Build history of the part. All positions in model axes, mm. Round coordinates to 2 decimals unless told otherwise and drop trailing zeros. Write each loop counter-clockwise with the first axis right and the second up, starting at its lowest first coordinate (ties: lowest second). Pieces come first, ordered by that corner, then holes. Notation, with made-up numbers: M -38.75,85.25 L -8.75,85.25 A18 cw -8.75,94.25 Z; hole C -28,3 d9. An arc over 180 degrees is marked long. Use a Markdown table: item, result.
Autodesk Inventor part; units mm, degrees
ref_plane "YZ Plane" through (0, 0, 0) normal (1, 0, 0) x (0, 1, 0)
ref_plane "XZ Plane" through (0, 0, 0) normal (0, 1, 0) x (-1, 0, 0)
ref_plane "XY Plane" through (0, 0, 0) normal (0, 0, 1) x (1, 0, 0)
sketch "Sketch1" plane through (0, 0, 0) normal (0, 0, 1) x (1, 0, 0)
  line L0 (0, 40) -> (0, 0)
  line L1 (0, 0) -> (6, 0)
  line L2 (6, 0) -> (6, 8)
  line L3 (6, 8) -> (22, 8)
  line L4 (22, 8) -> (22, 0)
  line L5 (22, 0) -> (28, 0)
  line L6 (28, 0) -> (28, 40)
  line L7 (28, 40) -> (0, 40)
  dimension "d0" = 6
  dimension "d1" = 6
  dimension "d2" = 16
  dimension "d3" = 40
  dimension "d4" = 8
extrude "Extrusion1" add sketch "Sketch1" against normal blind 8
sketch "Sketch2" plane through (28, 0, 0) normal (1, 0, 0) x (0, 0, -1)
  circle A0 centre (4, 4) radius 2
  line L0 (0, 0) -> (8, 0)
  line L1 (0, 0) -> (8, 0)
  point P0 (4, 0)
  dimension "d7" = 4
  dimension "d8" = 4
  dimension "d9" = 8
extrude "Extrusion2" cut sketch "Sketch2" against normal through all
fillet "Fillet1" radius 4 5 edges at (25, 0, 0) (3, 0, 0) (3, 0, -8) (25, 0, -8) (14, 8, -8)
sketch "Sketch3" plane through (0, 0, -8) normal (0, 0, -1) x (-1, 0, 0)
  line L0 (0, 40) -> (-28, 40)
  line L1 (-20, 40) -> (-16, 40)
  line L2 (-16, 40) -> (-16, 32)
  line L3 (-16, 32) -> (-20, 32)
  line L4 (-20, 32) -> (-20, 40)
  line L5 (-12, 40) -> (-8, 40)
  line L6 (-8, 40) -> (-8, 32)
  line L7 (-8, 32) -> (-12, 32)
  line L8 (-12, 32) -> (-12, 40)
  point P0 (0, 0)
  point P1 (-14, 40)
  dimension "d13" = 4
  dimension "d14" = 4
  dimension "d15" = 4
  dimension "d16" = 2
  dimension "d17" = 8
extrude "Extrusion3" add sketch "Sketch3" along normal blind 8
sketch "Sketch4" plane through (20, 32, -8) normal (1, 0, 0) x (0, 0, -1)
  circle A0 centre (4, 4) radius 2
  line L0 (8, 8) -> (8, 0)
  point P0 (-8, -32)
  dimension "d20" = 4
  dimension "d21" = 8
  dimension "d22" = 4
  dimension "d23" = 4
extrude "Extrusion4" cut sketch "Sketch4" against normal through all
fillet "Fillet2" radius 4 6 edges at (10, 40, -16) (18, 40, -16) (18, 32, -16) (10, 32, -16) (18, 32, -8) (10, 32, -8)
fillet "Fillet3" radius 4 4 edges at (14, 40, 0) (4, 40, -8) (14, 40, -8) (24, 40, -8)
sketch "Sketch5" plane through (0, 0, 0) normal (0, 0, 1) x (1, 0, 0)
  circle A0 centre (4, 34) radius 1.55
  line L0 (0, 36) -> (28, 36) construction
  line L1 (0, 36) -> (0, 4) construction
  circle A1 centre (4, 14) radius 1.55
  circle A2 centre (24, 34) radius 1.55
  circle A3 centre (24, 14) radius 1.55
  line L2 (28, 4) -> (28, 36) construction
  point P0 (0, 0)
  point P1 (14, 36)
  dimension "d30" = 20
  dimension "d33" = 20
  dimension "d36" = 2
  dimension "d37" = 10
  dimension "d38" = 3.1
extrude "Extrusion5" cut sketch "Sketch5" against normal up to surface (8 mm away)
equation "\"d0\" = d1"
equation "\"d4\" = 2 * arm_rod_diam"
equation "\"d5\" = 2 * arm_rod_diam"
equation "\"d7\" = arm_rod_diam"
equation "\"d8\" = 0.5 * d9"
equation "\"d12\" = arm_rod_diam"
equation "\"d13\" = d14"
equation "\"d18\" = 2 * arm_rod_diam"
equation "\"d20\" = arm_rod_diam"
equation "\"d22\" = 0.5 * d21"
equation "\"d23\" = d22"
equation "\"d26\" = arm_rod_diam"
equation "\"d27\" = arm_rod_diam"
equation "\"arm_rod_diam\" = 4"
properties part number "camera_arm"
Q1. Cut at D-D on z = -1. Give the cut face in (x, y).
Response values:
| item | result |
|---|---|
| outline | M 0,1.35 L 6,1.35 L 6,8 L 22,8 L 22,1.35 L 28,1.35 L 28,38.65 L 0,38.65 Z; hole C 4,14 d3.1; hole C 4,34 d3.1; hole C 24,14 d3.1; hole C 24,34 d3.1 |
Q2. Cut at B-B on y = 14. Give the cut face in (x, z).
Response values:
| item | result |
|---|---|
| outline | M 0,-8 L 2.45,-8 L 2.45,0 L 0,0 Z; M 5.55,-8 L 22.45,-8 L 22.45,0 L 5.55,0 Z; M 25.55,-8 L 28,-8 L 28,0 L 25.55,0 Z |
Q3. Drill centre lines: L1, parallel to Y at x = 10.85, z = -12; L2, parallel to X at y = 33, z = -1; L3, parallel to Z at x = 1, y = 12. Where is each one in solid material? Low to high.
Response values:
| item | result |
|---|---|
| L1 | y = 32 to 34, 38 to 40 |
| L2 | x = 0 to 2.82, 5.18 to 22.82, 25.18 to 28 |
| L3 | z = -8 to 0 |
Q4. Cut at A-A on x = 4. Count the separate pieces of the cut face and the enclosed holes in it, and give its area (3 significant figures).
Response values:
| item | result |
|---|---|
| separate pieces | 3 |
| enclosed holes | 1 |
| area | 244 mm2 |
Q5. Two-plate mould, pull along Z, no slides. Class faces 1 (the flat face through (8, 35, -10)), 2 (the cylindrical face through (25.042, 1.203, -1.141)), 3 (the cylindrical face through (3, 2.8, -2.4)), 4 (the cylindrical face through (3.944, 38.859, -6.797)): +Z half, -Z half, draft (parallel to the pull), parting line (faces both ways), or undercut.
Response values:
| item | result |
|---|---|
| face 1 | draft |
| face 2 | +Z half |
| face 3 | undercut |
| face 4 | -Z half |
Q6. Drop flat-ended pins along their axis: P1, Ø14, axis at x = 18.5, y = 26, coming from the -Z side; P2, Ø6, axis at x = 23.5, z = -10.5, coming from the +Y side; P3, Ø12, axis at x = 20.5, y = 21, coming from the -Z side. Give the stop position or say it passes through.
Response values:
| item | result |
|---|---|
| P1 | stops at z = -14.65 |
| P2 | stops at y = 37.94 |
| P3 | stops at z = -8 |
